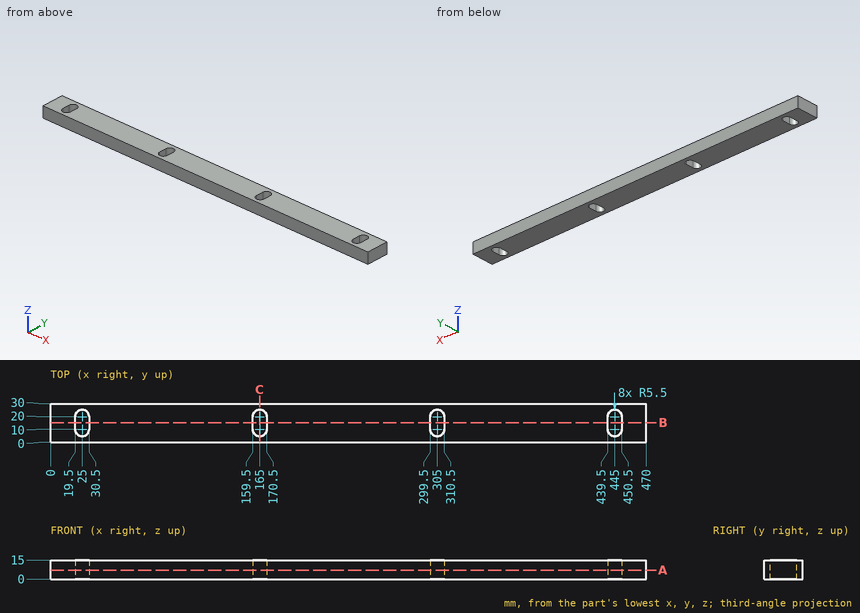
Geometry check sheet. Reference: drawing and pictorial views, mm from the part's lowest x, y, z. Round coordinates to 2 decimals unless told otherwise and drop trailing zeros. Loops run counter-clockwise (first coordinate to the right, second up) from the corner with the lowest first, then second, coordinate; pieces in that order, holes last. Notation, with made-up numbers: (42, 46) -> (52, 46) arc R26 cw to (52, 83) -> close; hole circle Ø8 at (23, 46.5). An arc over 180 degrees is marked (long way). Use a Markdown table: item, result.
(1) Sectioned sample at A-A (z = 7). Enter the section's corners in (x, y), then the cut area to 3 significant figures.
Calculated:
| item | result |
|---|---|
| outline | (0, 0) -> (470, 0) -> (470, 30) -> (0, 30) -> close; hole (19.5, 10) arc R5.5 ccw to (30.5, 10) -> (30.5, 20) arc R5.5 ccw to (19.5, 20) -> close; hole (159.5, 10) arc R5.5 ccw to (170.5, 10) -> (170.5, 20) arc R5.5 ccw to (159.5, 20) -> close; hole (299.5, 10) arc R5.5 ccw to (310.5, 10) -> (310.5, 20) arc R5.5 ccw to (299.5, 20) -> close; hole (439.5, 10) arc R5.5 ccw to (450.5, 10) -> (450.5, 20) arc R5.5 ccw to (439.5, 20) -> close |
| area | 13,300 mm² |
(2) Scan lines: probe 1 along X at (y, z) = (15.5, 3); probe 2 along X at (y, z) = (7, 4.5). Record each from-to range of solid material in increasing order.
Calculated:
| item | result |
|---|---|
| probe 1 | 0 to 19.5, 30.5 to 159.5, 170.5 to 299.5, 310.5 to 439.5, 450.5 to 470 |
| probe 2 | 0 to 20.39, 29.61 to 160.39, 169.61 to 300.39, 309.61 to 440.39, 449.61 to 470 |
(3) Sectioned sample at C-C (x = 165). Enter the section's corners in (y, z).
Calculated:
| item | result |
|---|---|
| outline | (0, 0) -> (4.5, 0) -> (4.5, 15) -> (0, 15) -> close; (25.5, 0) -> (30, 0) -> (30, 15) -> (25.5, 15) -> close |
(4) Go/stop test with a flat-tipped pin: P1, Ø6, axis at x = 81, z = 13, coming from the -Y side. Record where the tip stops, or that it passes through.
Calculated:
| item | result |
|---|---|
| P1 | y = 0 |
(5) Sectioned sample at B-B (y = 15.25). Enter the section's corners in (x, z), then the cut area to 3 significant figures.
Calculated:
| item | result |
|---|---|
| outline | (0, 0) -> (19.5, 0) -> (19.5, 15) -> (0, 15) -> close; (30.5, 0) -> (159.5, 0) -> (159.5, 15) -> (30.5, 15) -> close; (170.5, 0) -> (299.5, 0) -> (299.5, 15) -> (170.5, 15) -> close; (310.5, 0) -> (439.5, 0) -> (439.5, 15) -> (310.5, 15) -> close; (450.5, 0) -> (470, 0) -> (470, 15) -> (450.5, 15) -> close |
| area | 6,390 mm² |
